The listing builds one solid part. Answer for the finished solid, in the listing's coordinates (mm). A direction names the side the tool comes from. Coordinates: 2 decimals unless noted, no trailing zeros. Order: outer loops, then holes, each group sorted by start corner. A loop starts at its lowest first (then second) coordinate and runs counter-clockwise, first axis right, second up.
```python
from build123d import *

# Parameters (mm, degrees)
SKETCH_3_R               = 4
EXTRUDE_1_DEPTH          = 13
SKETCH_5_R               = 3.25
EXTRUDE_2_DEPTH          = 2
SKETCH_6_R               = 5
EXTRUDE_3_DEPTH          = 144
CHAMFER_2_SIZE           = 1
SKETCH_69_R              = 6
EXTRUDE_4_DEPTH          = 28
HOLE_WIZARD_1_D          = 8
HOLE_WIZARD_1_DEPTH      = 25
HOLE_WIZARD_1_TIP        = 2.403442476
CUT_EXTRUDE_1_DEPTH      = 28
CUT_EXTRUDE_1_DEPTH_BACK = 28
SKETCH_70_R              = 3


with BuildPart() as part:
    # Sketch 3 → Extrude 1 (new body)
    with BuildSketch(Plane(origin=(0, 0, 0), x_dir=(0, 0, -1), z_dir=(1, 0, 0))):
        Circle(SKETCH_3_R)
    extrude(amount=-EXTRUDE_1_DEPTH)

    # Sketch 5 → Extrude 2 (add)
    with BuildSketch(Plane.ZY.offset(13)):
        Circle(SKETCH_5_R)
    extrude(amount=EXTRUDE_2_DEPTH)

    # Sketch 6 → Extrude 3 (add)
    with BuildSketch(Plane.ZY.offset(15)):
        Circle(SKETCH_6_R)
    extrude(amount=EXTRUDE_3_DEPTH)

    # Chamfer 2
    chamfer_2_edges = [part.edges().sort_by_distance(p)[0] for p in [
        (0, 0, 4),
    ]]
    chamfer(chamfer_2_edges, length=CHAMFER_2_SIZE)

    # Sketch 69 → Extrude 4 (add)
    with BuildSketch(Plane.ZY.offset(159)):
        Circle(SKETCH_69_R)
    extrude(amount=EXTRUDE_4_DEPTH)

    # Hole Wizard 1
    with Locations(Plane.ZY.offset(187)):
        with Locations((0, 0)):
            Hole(HOLE_WIZARD_1_D / 2, depth=HOLE_WIZARD_1_DEPTH)
            with Locations((0, 0, -(HOLE_WIZARD_1_DEPTH + HOLE_WIZARD_1_TIP / 2))):  # 118° drill point
                Cone(0, HOLE_WIZARD_1_D / 2, HOLE_WIZARD_1_TIP, mode=Mode.SUBTRACT)

    # Sketch 70 → Cut-Extrude 1 (cut, two sides: drawn at the far end of the back side and taken through both)
    with BuildSketch(Plane.XY.offset(-CUT_EXTRUDE_1_DEPTH_BACK)):
        with Locations(Location((-167, 0, 0), (0, 0, 180))):
            Circle(SKETCH_70_R)
    extrude(amount=CUT_EXTRUDE_1_DEPTH + CUT_EXTRUDE_1_DEPTH_BACK, mode=Mode.SUBTRACT)


solid = part.part
```
(1) The mould has two halves that part along X. Classify faces 1 (the face through (0, 0, 0)), 2 (the face through (-6.916, -3.905, 0.867)), 3 (the face through (-169.86, -0.9, -4.35)): released by +X, released by -X, zero draft, split by the parting line, or undercut.
(2) Each of these flat-tipped pins is pushed along its axis until it touches: pin 1 Ø4 at (x, y) = (-64.5, 4) entering from -Z; pin 2 Ø1.5 at (x, z) = (-37.5, -4) entering from -Y; pin 3 Ø5 at (y, z) = (4.5, 4.5) entering from +X. Where does it stop, or does it pass through?
(3) Find section A-A (x = -167). Write down the section's boundary in (y, z), and give its area (3 significant figures).
(4) For faces 4 (the face through (-159, 4, -4)), 5 (the face through (-169.86, -0.9, 4.3)), 6 (the face through (-174, 0, 4)), 7 (the face through (-187, -3.92, -1.42)), 8 (the face through (-15, -3.3, 1)), determine the directions among +Z, -Z, +X, -X, +Y, -Y from which every point of the face is accessible in a straight line to the end or side of a thin tool.
(5) Consider line 1 (Y direction, x = -168.75, z = 0); line 2 (Z direction, x = -40.5, y = 4.25); line 3 (X direction, y = 4.75, z = 2.75). Determine where each line is inside the solid, lowest interval first.
(6) Find section B-B (x = -96.5). Write down the section's boundary in (y, z), and give its area (3 significant figures).
Findings below:
1. face 1: released by +X
1. face 2: zero draft
1. face 3: undercut
2. pin 1: stops at z = -4.58
2. pin 2: stops at y = -3.8
2. pin 3: stops at x = -0.86
3. outline: (-3, -5.2) - (-3, -2.65) arc R4 cw to (-3, 2.65) - (-3, 5.2) arc R6 ccw to start; (3, -5.2) arc R6 ccw to (3, 5.2) - (3, 2.65) arc R4 cw to (3, -2.65) - close
3. area: 37.0 mm2
4. face 4: +X
4. face 5: +Z, -Z
4. face 6: -X
4. face 7: +Z, -Z, -X, +Y, -Y
4. face 8: none
5. line 1: y = -6 to -4, 4 to 6
5. line 2: z = -2.63 to 2.63
5. line 3: x = -187 to -159
6. outline: circle Ø10 at (0, 0)
6. area: 78.5 mm2
